Autodesk Inventor part; units mm, degrees
ref_plane "YZ Plane" through (0, 0, 0) normal (1, 0, 0) x (0, 1, 0)
ref_plane "XZ Plane" through (0, 0, 0) normal (0, 1, 0) x (-1, 0, 0)
ref_plane "XY Plane" through (0, 0, 0) normal (0, 0, 1) x (1, 0, 0)
sketch "Sketch6" plane through (0, 0, 0) normal (0, 1, 0) x (-1, 0, 0)
  line L0 (0, 0) -> (40, 0)
  line L1 (40, 0) -> (40, 70)
  line L2 (40, 70) -> (0, 70)
  line L3 (0, 70) -> (0, 0)
  dimension "d10" = 40
  dimension "d11" = 70
extrude "Extrusion3" add sketch "Sketch6" along normal blind 25
shell "Shell1" thickness 1 removed faces 3 at (0, 8.3333, 46.6667) at (-40, 8.3333, 23.3333) at (-26.6667, 25, 23.3333)
sketch "Sketch7" plane through (-40, 0, 70) normal (0, 0, 1) x (1, 0, 0)
  line L0 (0, 25) -> (0, 1)
  line L1 (40, 0) -> (0, 0)
  line L2 (40, 1) -> (40, 25)
  circle A0 centre (20, 12.5) radius 3.5
  dimension "d15" = 7
extrude "Extrusion4" cut sketch "Sketch7" against normal blind 1
sketch "Sketch8" plane through (0, 0, 0) normal (0, -1, 0) x (1, 0, 0)
  line L0 (-40, 70) -> (0, 70)
  line L1 (0, 0) -> (-40, 0)
  circle A0 centre (-20, 35) radius 2
  dimension "d18" = 4
extrude "Extrusion5" cut sketch "Sketch8" against normal blind 1
properties part number "MAN_SERVO_HANDLER" material "ABS Plastic"
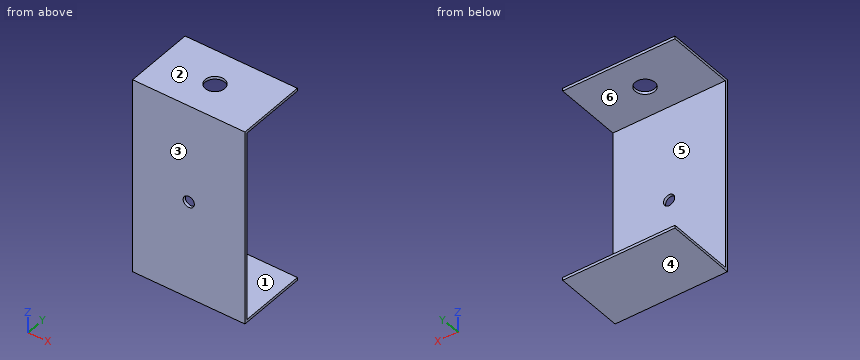
Here's how the part is built. I have some questions about the finished solid (model axes, mm). Face numbers are marked on the shaded views. A direction names the side the tool comes from. Give positions to 0.01 mm unless a question says otherwise; leave off trailing zeros. Order: outer loops, then holes, each group sorted by start corner. A loop starts at its lowest first (then second) coordinate and runs counter-clockwise, first axis right, second up. Notation, with made-up numbers: (57.5, 35.25) - (85.5, 35.25) arc R23 ccw to (85.5, 72.25) - close; hole circle Ø5 at (12, 81.25). An arc over 180 degrees is marked (long way). Answer as a JSON object with one key per item and string values. Group by question number.
Item 1: Which directions (+Z, -Z, +X, -X, +Y, -Y) give clear straight access to the entire face, cutting with the end or side of a thin tool? Please do the marked faces 1 and 2.
Item 2: If we section it at A-A on y = 12.5: Please give me the cut outline in (x, z), and give its area (3 significant figures).
Item 3: If we section it at C-C on z = 35: Please give me the cut outline in (x, y).
Item 4: If we section it at D-D on y = 7.75: Please give me the cut outline in (x, z), and give its area (3 significant figures).
Item 5: If we mould it in two halves opening along Z, with no side actions, what happens to the marked faces 3, 4, 5 and 6? For each: pulls with the +Z half, pulls with the -Z half, needs draft (parallel to the pull), parting line crosses it, or undercut.
Item 6: If we section it at B-B on x = -20: Please give me the cut outline in (y, z).
Item 7: Please list where these lines run through material, in increasing order: probe 1 along Z at (x, y) = (-30.5, 1.5); probe 2 along Z at (x, y) = (-20, 0.7); probe 3 along Y at (x, z) = (-20, 69.7).
Item 8: For P1, Ø1, axis at x = -34, y = 16, coming from the -Z side; P2, Ø12, axis at x = -4.5, z = 50.5, coming from the +Y side; P3, Ø6.5, axis at x = -20, y = 12.5, coming from the +Z side, each with a flat end and sliding along its axis, tell me the tip position at first contact or that it passes through.
Result set:
{
 "1": {"face 1": "+X, -X, +Y", "face 2": "+Z, +X, -X, +Y, -Y"},
 "2": {"outline": "(-40, 0) - (0, 0) - (0, 1) - (-40, 1) - close; (-40, 69) - (-23.5, 69) - (-23.5, 70) - (-40, 70) - close; (-16.5, 69) - (0, 69) - (0, 70) - (-16.5, 70) - close", "area": "73.0 mm²"},
 "3": {"outline": "(-40, 0) - (-22, 0) - (-22, 1) - (-40, 1) - close; (-18, 0) - (0, 0) - (0, 1) - (-18, 1) - close"},
 "4": {"outline": "(-40, 0) - (0, 0) - (0, 1) - (-40, 1) - close; (-40, 69) - (0, 69) - (0, 70) - (-40, 70) - close", "area": "80.0 mm²"},
 "5": {"face 3": "needs draft", "face 4": "pulls with the -Z half", "face 5": "undercut", "face 6": "undercut"},
 "6": {"outline": "(0, 0) - (25, 0) - (25, 1) - (1, 1) - (1, 33) - (0, 33) - close; (0, 37) - (1, 37) - (1, 69) - (9, 69) - (9, 70) - (0, 70) - close; (16, 69) - (25, 69) - (25, 70) - (16, 70) - close"},
 "7": {"probe 1": "0 to 1, 69 to 70", "probe 2": "0 to 33, 37 to 70", "probe 3": "0 to 9, 16 to 25"},
 "8": {"P1": "z = 0", "P2": "y = 1", "P3": "z = 1"}
}
